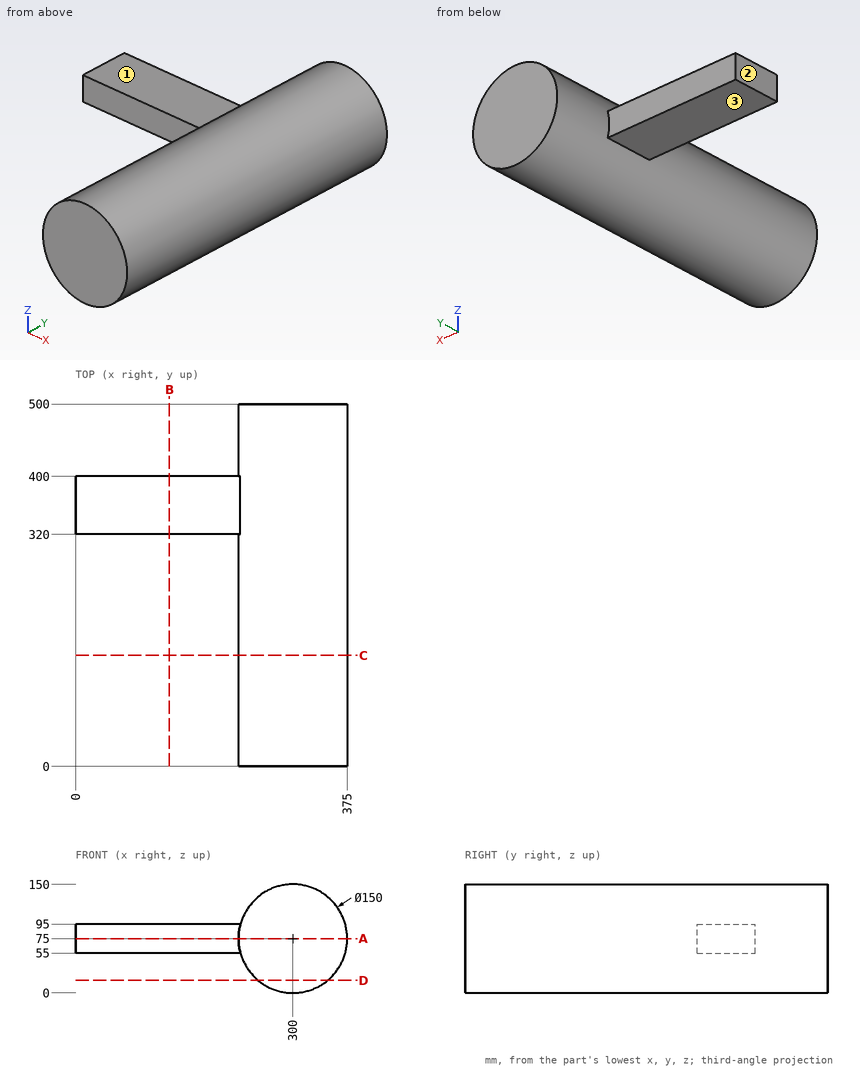
The drawing under review shows one solid part. Ordinate dimensions are in mm from its lowest x, y, z. A direction names the side the tool comes from. Give positions to 0.01 mm unless a question says otherwise; leave off trailing zeros. Write each loop counter-clockwise with the first axis right and the second up, starting at its lowest first coordinate (ties: lowest second). Pieces come first, ordered by that corner, then holes.
1. Tool access review of the marked faces 1, 2 and 3: name each direction out of +Z, -Z, +X, -X, +Y, -Y from which nothing blocks a thin tool from reaching the whole face with its end or side.
2. Add section C-C, the plane y = 153. Write out the cut boundary in (x, z), plus the area to 3 significant figures.
3. Add section B-B, the plane x = 129.5. Write out the cut boundary in (y, z), plus the area to 3 significant figures.
4. Wall thickness on L1, parallel to Z at x = 158.5, y = 332; L2, parallel to X at y = 102.5, z = 74; L3, parallel to Z at x = 301, y = 291.5: over which ranges is each line inside the solid? List them lowest first.
5. Add section D-D, the plane z = 17.5. Write out the cut boundary in (x, y).
6. Add section A-A, the plane z = 75. Write out the cut boundary in (x, y).
7. For P1, Ø1.5, axis at x = 83.5, y = 362.5, coming from the +Z side; P2, Ø20, axis at x = 111, z = 79.5, coming from the +Y side; P3, Ø10, axis at y = 384, z = 118, coming from the +X side, all flat-tipped, find the tip position at first contact; note any pin that passes through.
Worked answers:
1. face 1: +Z, -X, +Y, -Y
1. face 2: +Z, -Z, -X, +Y, -Y
1. face 3: -Z, -X, +Y, -Y
2. outline: circle Ø150 at (300, 75)
2. area: 17,700 mm2
3. outline: (320, 55) - (400, 55) - (400, 95) - (320, 95) - close
3. area: 3,200 mm2
4. L1: z = 55 to 95
4. L2: x = 225.01 to 374.99
4. L3: z = 0.01 to 149.99
5. outline: (251.85, 0) - (348.15, 0) - (348.15, 500) - (251.85, 500) - close
6. outline: (0, 320) - (225, 320) - (225, 0) - (375, 0) - (375, 500) - (225, 500) - (225, 400) - (0, 400) - close
7. P1: stops at z = 95
7. P2: stops at y = 400
7. P3: stops at x = 364.66
